Part model, mm, in its own coordinate system. Face numbers are marked on the shaded views. A direction names the side the tool comes from. Give positions to 0.01 mm unless a question says otherwise; leave off trailing zeros. Order: outer loops, then holes, each group sorted by start corner. A loop starts at its lowest first (then second) coordinate and runs counter-clockwise, first axis right, second up. Notation, with made-up numbers: (-3.75, 10) -> (4.25, 10) arc R12 ccw to (4.25, 24) -> close; hole circle Ø1 at (9, -33). An arc over 180 degrees is marked (long way). Write item = value, one per line. Start each with the question number.
(1) Two-plate mould, pull along X, no slides. Class the marked faces 6 and 7: pulls with the +X half, pulls with the -X half, needs draft (parallel to the pull), parting line crosses it, or undercut.
(2) Saw through at A-A, the plane x = 107. List the corners of the cut face in (y, z).
(3) Which spindle directions (+Z, -Z, +X, -X, +Y, -Y) get a long thin tool onto all of the face, cutting with end or side? Do the marked faces 1, 2, 3, 4 and 5. Say none if no direction does.
(4) Probe line 1 along Y through (x, z) = (432, -185.5); line 2 along Y through (x, z) = (55.5, 33); line 3 along Z through (x, y) = (-305, 414.5). List the from-to ranges inside material, lowest first. Write a range as from..to.
(5) Saw through at B-B, the plane y = 330. List the corners of the cut face in (x, z).
(6) Flat gauge pins, fed straight in: pin 1 (9 mm diameter, centred on y = 427.5, z = -27.5, fed in from -X); pin 2 (3 mm diameter, centred on y = 103.5, z = 191, fed in from -X); pin 3 (1 mm diameter, centred on x = -192.5, z = -101, fed in from -Y). Where does each tip first touch, or does it go through?
(7) Saw through at C-C, the plane z = 102. List the corners of the cut face in (x, y), then the cut area to 3 significant figures.
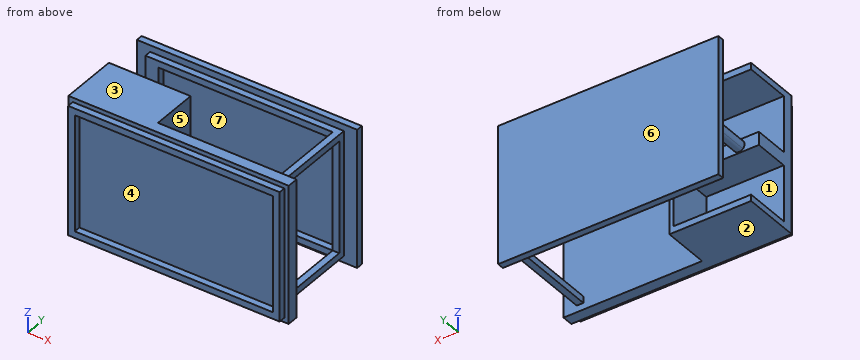
from build123d import *

# Parameters (mm, degrees)
SKETCH1_W           = 1000
SKETCH1_H           = 628
BOSS_EXTRUDE1_DEPTH = 50
SKETCH2_W           = 371
SKETCH2_H           = 628
BOSS_EXTRUDE2_DEPTH = 210
SKETCH3_W           = 569
SKETCH3_H           = 210
CUT_EXTRUDE1_DEPTH  = 352
BOSS_EXTRUDE3_DEPTH = 160
SKETCH6_W           = 628
SKETCH6_H           = 30
BOSS_EXTRUDE4_DEPTH = 1000
BOSS_EXTRUDE5_DEPTH = 242
BOSS_EXTRUDE6_START = 30
SKETCH8_W           = 790
SKETCH8_H           = 30
SKETCH8_R           = 25
BOSS_EXTRUDE6_DEPTH = 30
SKETCH9_W           = 30
SKETCH9_H           = 30
BOSS_EXTRUDE7_DEPTH = 388
SKETCH10_W          = 900
SKETCH10_H          = 30
BOSS_EXTRUDE8_DEPTH = 30


with BuildPart() as part:
    # Sketch1 → Boss-Extrude1 (new body)
    with BuildSketch(Plane(origin=(0, 0, 0), x_dir=(1, 0, 0), z_dir=(0, 1, 0))):
        Rectangle(SKETCH1_W, SKETCH1_H)
    extrude(amount=BOSS_EXTRUDE1_DEPTH)

    # Sketch2 → Boss-Extrude2 (add)
    with BuildSketch(Plane(origin=(0, 50, 0), x_dir=(1, 0, 0), z_dir=(0, 1, 0))):
        with Locations((-314.5, 0)):
            Rectangle(SKETCH2_W, SKETCH2_H)
    extrude(amount=BOSS_EXTRUDE2_DEPTH)

    # Sketch3 → Cut-Extrude1 (cut)
    with BuildSketch(Plane.ZY.offset(500)):
        with Locations((-0.5, 155)):
            Rectangle(SKETCH3_W, SKETCH3_H)
    extrude(amount=-CUT_EXTRUDE1_DEPTH, mode=Mode.SUBTRACT)

    # Sketch4 → Boss-Extrude3 (add)
    with BuildSketch(Plane(origin=(0, 50, 0), x_dir=(1, 0, 0), z_dir=(0, 1, 0))):
        Polygon((-342.55887522, -29.5), (-324, 0.5), (-342.55887522, 30.5), (-500, 30.5), (-500, -29.5), align=None)
        Polygon((-148, 30.5), (-305.44112478, 30.5), (-324, 0.5), (-305.44112478, -29.5), (-148, -29.5), align=None)
        Polygon((-305.44112478, -29.5), (-324, 0.5), (-324, -29.5), align=None)
        Polygon((-324, -29.5), (-324, 0.5), (-342.55887522, -29.5), align=None)
        Polygon((-324, 0.5), (-305.44112478, 30.5), (-324, 30.5), align=None)
        Polygon((-342.55887522, 30.5), (-324, 0.5), (-324, 30.5), align=None)
    extrude(amount=BOSS_EXTRUDE3_DEPTH)



with BuildPart() as body_2:
    # Sketch6 → Boss-Extrude4 (new body)
    with BuildSketch(Plane(origin=(500, 0, 0), x_dir=(0, 0, -1), z_dir=(1, 0, 0))):
        with Locations((0, 455)):
            Rectangle(SKETCH6_W, SKETCH6_H)
    extrude(amount=-BOSS_EXTRUDE4_DEPTH)


with BuildPart() as part_1:
    add(part.part)

    add(body_2.part)  # Boss-Extrude5 merges body 2
    # Sketch7 → Boss-Extrude5 (add)
    with BuildSketch(Plane(origin=(0, 210, 0), x_dir=(1, 0, 0), z_dir=(0, 1, 0))):
        with BuildLine():
            ThreePointArc((-392.32233047, 18.17766953), (-410, 25.5), (-427.67766953, 18.17766953))
            Line((-427.67766953, 18.17766953), (-410, 0.5))
            Line((-410, 0.5), (-392.32233047, 18.17766953))
        make_face()
        with BuildLine():
            Line((-410, 0.5), (-427.67766953, 18.17766953))
            ThreePointArc((-427.67766953, 18.17766953), (-435, 0.5), (-427.67766953, -17.17766953))
            Line((-427.67766953, -17.17766953), (-410, 0.5))
        make_face()
        with BuildLine():
            Line((-410, 0.5), (-427.67766953, -17.17766953))
            ThreePointArc((-427.67766953, -17.17766953), (-410, -24.5), (-392.32233047, -17.17766953))
            Line((-392.32233047, -17.17766953), (-410, 0.5))
        make_face()
        with BuildLine():
            ThreePointArc((-385, 0.5), (-386.903011687, 10.067085809), (-392.32233047, 18.17766953))
            Line((-392.32233047, 18.17766953), (-410, 0.5))
            Line((-410, 0.5), (-392.32233047, -17.17766953))
            ThreePointArc((-392.32233047, -17.17766953), (-386.903011687, -9.067085809), (-385, 0.5))
        make_face()
    extrude(amount=BOSS_EXTRUDE5_DEPTH)

    # Sketch8 → Boss-Extrude6 (add)
    # profile 1 of 4: a face of its own
    with BuildSketch(Plane(origin=(0, 440, 0), x_dir=(-1, 0, 0), z_dir=(0, -1, 0)).offset(BOSS_EXTRUDE6_START)):
        Polygon((-440, -284), (-410, -284), (-410, -254), (-410, 254), (-410, 284), (-440, 284), align=None)
    # profile 2 of 4: a face of its own
    with BuildSketch(Plane(origin=(0, 440, 0), x_dir=(-1, 0, 0), z_dir=(0, -1, 0)).offset(BOSS_EXTRUDE6_START)):
        Polygon((-410, -284), (440, -284), (440, -254), (380, -254), (-410, -254), align=None)
    # profile 3 of 4: a face of its own
    with BuildSketch(Plane(origin=(0, 440, 0), x_dir=(-1, 0, 0), z_dir=(0, -1, 0)).offset(BOSS_EXTRUDE6_START)):
        with Locations((-15, 269)):
            Rectangle(SKETCH8_W, SKETCH8_H)
    # profile 4 of 4: a face of its own
    with BuildSketch(Plane(origin=(0, 440, 0), x_dir=(-1, 0, 0), z_dir=(0, -1, 0)).offset(BOSS_EXTRUDE6_START)):
        Polygon((380, -254), (440, -254), (440, 284), (380, 284), (380, 254), align=None)
        with Locations(Location((410, 0.5, 0), (0, 0, 90))):
            Circle(SKETCH8_R, mode=Mode.SUBTRACT)
    extrude(amount=-BOSS_EXTRUDE6_DEPTH)

    # Sketch9 → Boss-Extrude7 (add)
    with BuildSketch(Plane(origin=(0, 410, 0), x_dir=(-1, 0, 0), z_dir=(0, -1, 0))):
        with Locations((-425, -269)):
            Rectangle(SKETCH9_W, SKETCH9_H)
        with Locations((-425, 269)):
            Rectangle(SKETCH9_W, SKETCH9_H)
    extrude(amount=BOSS_EXTRUDE7_DEPTH)

    # Sketch10 → Boss-Extrude8 (add)
    with BuildSketch(Plane(origin=(0, 0, 0), x_dir=(-1, 0, 0), z_dir=(0, -1, 0))):
        Polygon((480, -294), (480, 264), (450, 264), (450, -264), (450, -294), align=None)
        Polygon((480, 264), (480, 294), (-480, 294), (-480, 264), (-450, 264), (450, 264), align=None)
        with Locations((0, -279)):
            Rectangle(SKETCH10_W, SKETCH10_H)
        Polygon((-450, 264), (-480, 264), (-480, -294), (-450, -294), (-450, -264), align=None)
    extrude(amount=BOSS_EXTRUDE8_DEPTH)


solid = part_1.part
Results list:
q1.face_6 = needs draft
q1.face_7 = undercut
q2.outline = (-30, -294) -> (0, -294) -> (0, -314) -> (50, -314) -> (50, 314) -> (0, 314) -> (0, 294) -> (-30, 294) -> (-30, 264) -> (0, 264) -> (0, -264) -> (-30, -264) -> close; (410, -284) -> (440, -284) -> (440, -314) -> (470, -314) -> (470, 314) -> (440, 314) -> (440, 284) -> (410, 284) -> (410, 254) -> (440, 254) -> (440, -254) -> (410, -254) -> close
q3.face_1 = -X
q3.face_2 = -Z, +X, -X, +Y, -Y
q3.face_3 = +Z, +X, -X, +Y, -Y
q3.face_4 = -Y
q3.face_5 = +Z, -Z
q4.line_1 = 0..50, 410..470
q4.line_2 = 0..50, 440..470
q4.line_3 = -284..-254, 254..284
q5.outline = circle Ø50 at (-410, -0.5); (410, -284) -> (440, -284) -> (440, -254) -> (410, -254) -> close; (410, 254) -> (440, 254) -> (440, 284) -> (410, 284) -> close
q6.pin_1 = -440
q6.pin_2 = -148
q6.pin_3 = 0
q7.outline = (-500, 0) -> (-480, 0) -> (-480, -30) -> (-450, -30) -> (-450, 0) -> (450, 0) -> (450, -30) -> (480, -30) -> (480, 0) -> (500, 0) -> (500, 50) -> (-129, 50) -> (-129, 260) -> (-148, 260) -> (-148, 50) -> (-500, 50) -> close; (-500, 440) -> (-440, 440) -> (-440, 410) -> (-380, 410) -> (-380, 440) -> (410, 440) -> (410, 410) -> (440, 410) -> (440, 440) -> (500, 440) -> (500, 470) -> (-500, 470) -> close
q7.area = 88,500 mm^2
